Geometry check sheet. Reference: the model listing, model coordinates, mm. A direction names the side the tool comes from. Round coordinates to 2 decimals unless told otherwise and drop trailing zeros. Write each loop counter-clockwise with the first axis right and the second up, starting at its lowest first coordinate (ties: lowest second). Pieces come first, ordered by that corner, then holes. Notation, with made-up numbers: M 31,27.5 L 44,27.5 A30 cw 44,55.5 Z; hole C 70,75 d11. An arc over 180 degrees is marked long. Put each result on its own line as item: value. Start each with the question number.
(1) Section check C-C on y = 19. Record the cut outline in (x, z), then the cut area to 3 significant figures.
(2) Mould release check, pull along Y, two halves, no side actions. Record for faces 1 (the flat face through (20, 47, 5)), 2 (the cylindrical face through (40.67, 27.6, 4.91)), 3 (the flat face through (20, 0, 5)): pulls with the +Y half, pulls with the -Y half, needs draft (parallel to the pull), parting line crosses it, or undercut.
(3) Material ranges on probe 1 along Y at (x, z) = (35, 2); probe 2 along Z at (x, y) = (30, 44.5); probe 3 along X at (y, z) = (5.5, 6.5), recorded low to high.
(4) Section check B-B on z = 4. Count the separate pieces of the cut face and the enclosed holes in it, then the cut area to 3 significant figures.
(5) Tool access check on faces 4 (the flat face through (40, 10, 5)), 5 (the flat face through (37, 25, 5)), 6 (the flat face through (40.3, 35, 4.9)), 7 (the flat face through (20, 25, 10)). Record the directions out of +Z, -Z, +X, -X, +Y, -Y that give a thin tool (end or side, any length) a straight path to the whole face; none if there is none.
(6) Gauge pin test, flat ends, axial feed: pin 1 (2 mm diameter, centred on x = 14.5, z = 2.5, fed in from -Y); pin 2 (10 mm diameter, centred on x = 31.5, y = 16, fed in from +Z); pin 3 (0.8 mm diameter, centred on x = 38, y = 12, fed in from -Z); pin 4 (1.2 mm diameter, centred on y = 18.5, z = 4.5, fed in from +X). Record the tip position at first contact, or that the pin passes through.
(7) Section check D-D on y = 33. Record the cut outline in (x, z).
(8) Section check A-A on x = 10. Record the cut outline in (y, z), then the cut area to 3 significant figures.
from build123d import *

# Parameters (mm, degrees)
SKETCH1_W           = 40
SKETCH1_H           = 50
BOSS_EXTRUDE1_DEPTH = 10
SHELL4_T            = 3
BOSS_EXTRUDE4_START = -15
SKETCH4_R           = 2
BOSS_EXTRUDE4_DEPTH = 15
SKETCH9_R           = 0.5
CUT_EXTRUDE2_DEPTH  = 5


with BuildPart() as part:
    # Sketch1 → Boss-Extrude1 (new body)
    with BuildSketch(Plane.XY):
        with Locations((20, 25)):
            Rectangle(SKETCH1_W, SKETCH1_H)
    extrude(amount=BOSS_EXTRUDE1_DEPTH)

    # Shell4 (no face opened: a closed hollow body)
    add(offset(amount=-SHELL4_T, mode=Mode.PRIVATE), mode=Mode.SUBTRACT)

    # Sketch4 → Boss-Extrude4 (add)
    with BuildSketch(Plane(origin=(0, 50, 0), x_dir=(1, 0, 0), z_dir=(0, 1, 0)).offset(BOSS_EXTRUDE4_START)):
        with BuildLine():
            Line((40, 0), (40.33712564, 0))
            ThreePointArc((40.33712564, 0), (45.339222659, -5.002097019), (40.33712564, -10.004194037))
            Line((40.33712564, -10.004194037), (40, -10))
            Line((40, -10), (40, 0))
        make_face()
        with Locations((42.669611329, -5.001048509)):
            Circle(SKETCH4_R, mode=Mode.SUBTRACT)
    extrude(amount=-BOSS_EXTRUDE4_DEPTH)

    # Sketch9 → Cut-Extrude2 (cut)
    with BuildSketch(Plane(origin=(0, 0, 0), x_dir=(-1, 0, 0), z_dir=(0, 0, -1))):
        with Locations((-38, 15)):
            Circle(SKETCH9_R)
        with Locations((-35, 15)):
            Circle(SKETCH9_R)
        with Locations((-32, 15)):
            Circle(SKETCH9_R)
        with Locations((-29, 15)):
            Circle(SKETCH9_R)
        with Locations((-26, 15)):
            Circle(SKETCH9_R)
        with Locations((-35, 12)):
            Circle(SKETCH9_R)
        with Locations((-32, 12)):
            Circle(SKETCH9_R)
        with Locations((-29, 12)):
            Circle(SKETCH9_R)
        with Locations((-26, 12)):
            Circle(SKETCH9_R)
        with Locations((-35, 9)):
            Circle(SKETCH9_R)
        with Locations((-32, 9)):
            Circle(SKETCH9_R)
        with Locations((-29, 9)):
            Circle(SKETCH9_R)
        with Locations((-26, 9)):
            Circle(SKETCH9_R)
        with Locations((-35, 6)):
            Circle(SKETCH9_R)
        with Locations((-32, 6)):
            Circle(SKETCH9_R)
        with Locations((-29, 6)):
            Circle(SKETCH9_R)
        with Locations((-26, 6)):
            Circle(SKETCH9_R)
        with Locations((-35, 3)):
            Circle(SKETCH9_R)
        with Locations((-32, 3)):
            Circle(SKETCH9_R)
        with Locations((-29, 3)):
            Circle(SKETCH9_R)
        with Locations((-26, 3)):
            Circle(SKETCH9_R)
        with Locations((-38, 12)):
            Circle(SKETCH9_R)
        with Locations((-38, 9)):
            Circle(SKETCH9_R)
        with Locations((-38, 6)):
            Circle(SKETCH9_R)
        with Locations((-38, 3)):
            Circle(SKETCH9_R)
    extrude(amount=-CUT_EXTRUDE2_DEPTH, mode=Mode.SUBTRACT)


solid = part.part
Answers follow:
1. outline: M 0,0 L 40,0 L 40,10 L 0,10 Z; hole M 3,3 L 37,3 L 37,7 L 3,7 Z
1. area: 264 mm^2
2. face 1: undercut
2. face 2: needs draft
2. face 3: pulls with the -Y half
3. probe 1: y = 0 to 2.5, 3.5 to 5.5, 6.5 to 8.5, 9.5 to 11.5, 12.5 to 14.5, 15.5 to 50
3. probe 2: z = 0 to 3, 7 to 10
3. probe 3: x = 0 to 3, 37 to 40
4. separate pieces: 2
4. enclosed holes: 6
4. area: 525 mm^2
5. face 4: +Z, -Z, +X, -Y
5. face 5: none
5. face 6: +Z, -Z, +X, +Y
5. face 7: +Z, +X, -X, +Y, -Y
6. pin 1: stops at y = 0
6. pin 2: stops at z = 10
6. pin 3: stops at z = 5
6. pin 4: stops at x = 40
7. outline: M 0,0 L 40.34,0 A5 ccw 40.34,10 L 40,10 L 0,10 Z; hole M 3,3 L 37,3 L 37,7 L 3,7 Z; hole C 42.67,5 d4
8. outline: M 0,0 L 50,0 L 50,10 L 0,10 Z; hole M 3,3 L 47,3 L 47,7 L 3,7 Z
8. area: 324 mm^2
